Geometry: see drawing. Coordinates: mm, zero at the bounding-box minimum. A direction names the side the tool comes from. Coordinates: 2 decimals unless noted, no trailing zeros. Write each loop counter-clockwise with the first axis right and the second up, starting at its lowest first coordinate (ties: lowest second). Pieces come first, ordered by that corner, then holes. Notation, with made-up numbers: M 81,55 L 108,55 A22 cw 108,93 Z; hole C 87.25,88.25 d10. An arc over 180 degrees is marked long. One line per item, written item: value. Start each with the question number.
Item 1: Pin query (flat end, axial travel): P1, Ø1, axis at x = 0.5, z = 6.5, coming from the +Y side; P2, Ø2.5, axis at y = 4, z = 3, coming from the -X side; P3, Ø5, axis at y = 2, z = 13, coming from the -X side; P4, Ø0.5, axis at x = 1, y = 1, coming from the +Z side. Return the tip coordinate at first contact, or that it passes through.
Item 2: Ray query, L1, parallel to Y at x = 1.25, z = 3.5; L2, parallel to Y at x = 1, z = 16.75; L3, parallel to Z at x = 0.9, y = 5.25. Return the intervals inside material, ascending. Write a range as from..to.
Item 3: Cut plane A-A, the plane y = 5. Output: boundary loops of the cut face in (x, z).
Item 4: Cut plane C-C, the plane x = 0.95. Output: boundary loops of the cut face in (y, z).
Item 5: Set-up query: the marked faces 1 and 2. Return all of +Z, -Z, +X, -X, +Y, -Y with unobstructed straight access to the full face (end or side cutting, diameter ignored); none if empty.
Item 6: Cut plane B-B, the plane z = 2.5. Output: boundary loops of the cut face in (x, y).
Item 7: Cut plane D-D, the plane y = 9.5. Output: boundary loops of the cut face in (x, z).
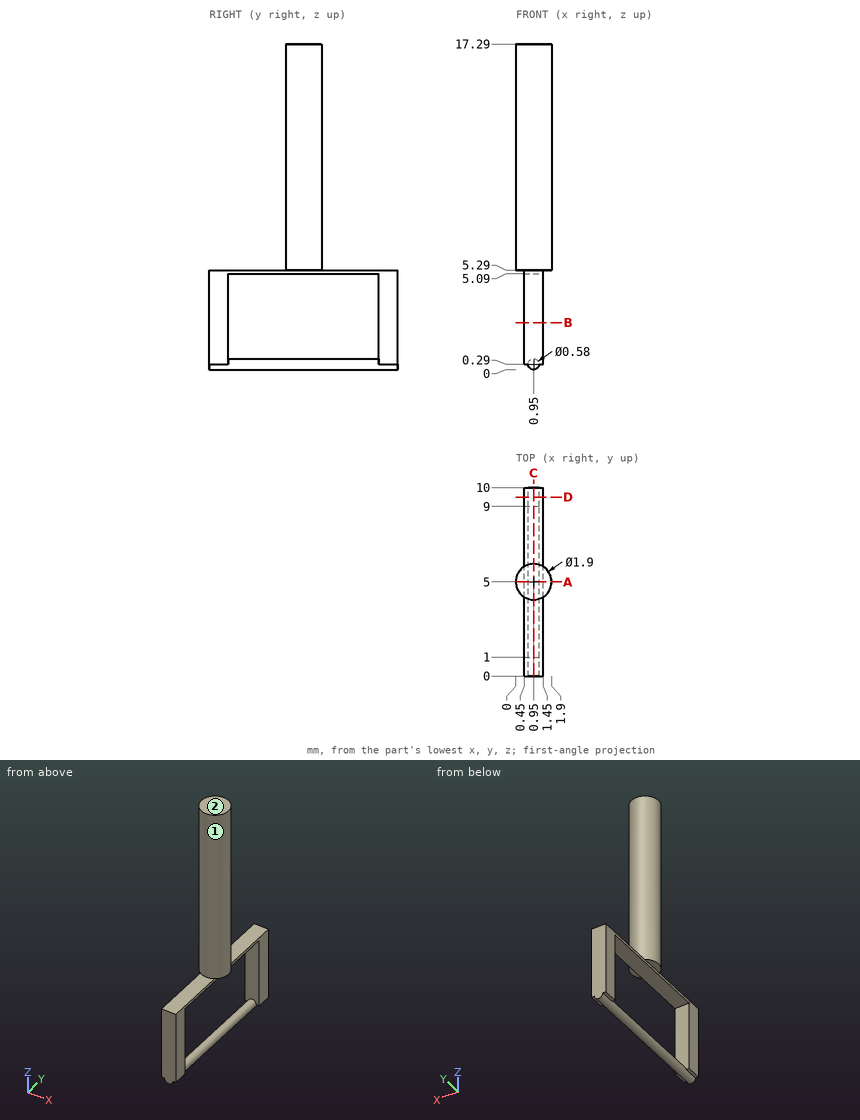
From the geometry:
1. P1: stops at y = 5.95
1. P2: passes through
1. P3: stops at x = 0.14
1. P4: stops at z = 5.29
2. L1: y = 0..1, 9..10
2. L2: y = 4.05..5.95
2. L3: z = 0..0.58, 5.09..17.29
3. outline: M 0,5.29 L 0.45,5.29 L 0.45,5.09 L 1.45,5.09 L 1.45,5.29 L 1.9,5.29 L 1.9,17.29 L 0,17.29 Z; C 0.95,0.29 d0.58
4. outline: M 0,0 L 10,0 L 10,5.29 L 5.95,5.29 L 5.95,17.29 L 4.05,17.29 L 4.05,5.29 L 0,5.29 Z; hole M 1,0.58 L 9,0.58 L 9,5.09 L 1,5.09 Z
5. face 1: +Z
5. face 2: +Z, +X, -X, +Y, -Y
6. outline: M 0.45,0 L 1.45,0 L 1.45,1 L 0.45,1 Z; M 0.45,9 L 1.45,9 L 1.45,10 L 0.45,10 Z
7. outline: M 0.45,0.29 L 0.66,0.29 A0.29 ccw 1.24,0.29 L 1.45,0.29 L 1.45,5.29 L 0.45,5.29 Z
